Read the model definition and answer for the solid it produces. Units are mm, in the model's axes. A direction names the side the tool comes from. Give positions to 0.01 mm unless a question says otherwise; leave off trailing zeros. Order: outer loops, then holes, each group sorted by start corner. A loop starts at its lowest first (then second) coordinate and runs counter-clockwise, first axis right, second up.
```python
from build123d import *

# Parameters (mm, degrees)
F1_DEPTH = 304.8
F3_DEPTH = 19.05
F5_DEPTH = 19.05


with BuildPart() as f1:
    # F0 (on Top) → F1 (new body)
    with BuildSketch(Plane.XY):
        Polygon((6.35, 0), (0, 0), (0, -9.525), (-4.7625, -9.525), (-4.7625, -19.05), (0, -31.75), (6.35, -31.75), (11.1125, -19.05), (11.1125, -9.525), (6.35, -9.525), align=None)
    extrude(amount=F1_DEPTH)

    # F2 (on face) → F3 (join)
    with BuildSketch(Plane(origin=(0, 0, 0), x_dir=(1, 0, 0), z_dir=(0, 0, -1))):
        Polygon((6.35, 9.525), (6.35, 19.05), (0, 19.05), (0, 9.525), (0, 0), (6.35, 0), align=None)
    extrude(amount=F3_DEPTH)

    # F4 (on face) → F5 (join)
    with BuildSketch(Plane.XY.offset(304.8)):
        Polygon((0, 0), (0, -9.525), (0, -19.05), (6.35, -19.05), (6.35, -9.525), (6.35, 0), align=None)
    extrude(amount=F5_DEPTH)


solid = f1.part
```
1) The part is cut by section C-C on y = -26.5. Determine the outline of the cut face in (x, z), and give its area (3 significant figures).
Final values:
outline: (-1.97, 0) - (8.32, 0) - (8.32, 304.8) - (-1.97, 304.8) - close
area: 3,140 mm2
2) Given pin 1 (3 mm diameter, centred on y = -22.5, z = 29.5, fed in from +X); pin 2 (2.5 mm diameter, centred on x = 9.5, z = 173, fed in from +Y) (3 decimals); pin 3 (6 mm diameter, centred on y = -22.5, z = 153, fed in from +X), each flat-ended and moving along its own axis, determine where each tip first touches the part or whether it passes through.
Final values:
pin 1: stops at x = 10.38
pin 2: stops at y = -9.525
pin 3: stops at x = 10.94
3) Consider L1, parallel to Z at x = -1.25, y = -16.5; L2, parallel to X at y = -1, z = 56; L3, parallel to X at y = -27.5, z = 271. Determine where each line is inside the solid, lowest interval first.
Final values:
L1: z = 0 to 304.8
L2: x = 0 to 6.35
L3: x = -1.59 to 7.94
4) For a pull along Z with two mould halves and no side action, classify faces 1 (the face through (3, -9, 323.85)), 2 (the face through (3, -10, -19.05)), 3 (the face through (11.112, -14, 150)) as released by +Z, released by -Z, zero draft, split by the parting line, or undercut.
Final values:
face 1: released by +Z
face 2: released by -Z
face 3: zero draft
5) The part is cut by section B-B on y = -3. Determine the outline of the cut face in (x, z).
Final values:
outline: (0, -19.05) - (6.35, -19.05) - (6.35, 323.85) - (0, 323.85) - close
6) A tool of negligible diameter and unlimited length cuts with its end or side. For faces 4 (the face through (3, -31.75, 150)), 5 (the face through (3, -19.05, -9)), 6 (the face through (3, -19.05, 314)), from which of +Z, -Z, +X, -X, +Y, -Y can it reach the whole face along a straight path? Write none if from no direction.
Final values:
face 4: +Z, -Z, +X, -X, -Y
face 5: -Z, +X, -X, -Y
face 6: +Z, +X, -X, -Y
